Check sheet for the modelled part. Datum: model origin and axes. Units: mm. Face numbers are marked on the shaded views. Give positions to 0.01 mm unless a question says otherwise; leave off trailing zeros. Order: outer loops, then holes, each group sorted by start corner. A loop starts at its lowest first (then second) coordinate and runs counter-clockwise, first axis right, second up. Notation, with made-up numbers: (78, -23.75) -> (82, -23.75) arc R24 ccw to (82, 8.25) -> close; hole circle Ø1 at (22, 44.5). An arc over 180 degrees is marked (long way). Write each question's results on one line, items separated by ' | '.
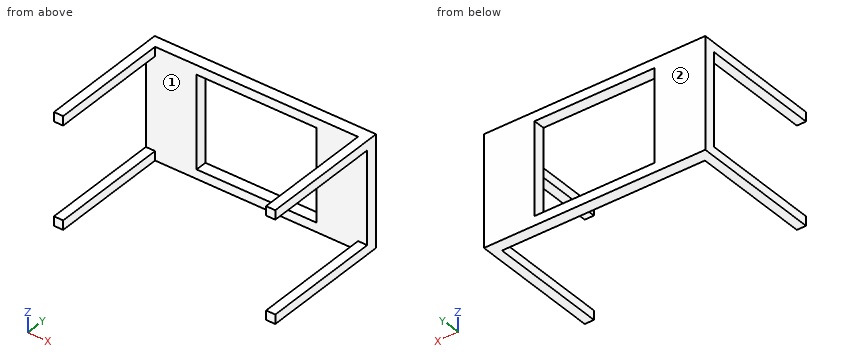
from build123d import *

# Parameters (mm, degrees)
F0_W     = 1219.2
F0_H     = 609.6
F1_DEPTH = 63.5
F2_W     = 660.4
F2_H     = 508
F3_DEPTH = 114.3
F4_W     = 50.8
F4_H     = 50.8
F5_DEPTH = 660.4


with BuildPart() as f1:
    # F0 (on Front) → F1 (new body)
    with BuildSketch(Plane.XZ):
        with Locations((-609.6, 304.8)):
            Rectangle(F0_W, F0_H)
    extrude(amount=F1_DEPTH)

    # F2 (on face) → F3 (cut)
    with BuildSketch(Plane.XZ.offset(63.5)):
        with Locations((-609.6, 304.8)):
            Rectangle(F2_W, F2_H)
    extrude(amount=-F3_DEPTH, mode=Mode.SUBTRACT)

    # F4 (on face) → F5 (join)
    with BuildSketch(Plane.XZ.offset(63.5)):
        with Locations((-1193.8, 584.2)):
            Rectangle(F4_W, F4_H)
        with Locations((-1193.8, 25.4)):
            Rectangle(F4_W, F4_H)
        with Locations((-25.4, 25.4)):
            Rectangle(F4_W, F4_H)
        with Locations((-25.4, 584.2)):
            Rectangle(F4_W, F4_H)
    extrude(amount=F5_DEPTH)


solid = f1.part
1. Gauge pin test, flat ends, axial feed: pin 1 Ø19 at (y, z) = (-36.5, 301.5) entering from +X; pin 2 Ø8 at (x, z) = (-976, 161) entering from -Y. Record the tip position at first contact, or that the pin passes through.
Verdict:
pin 1: stops at x = 0 | pin 2: stops at y = -63.5
2. Section check D-D on x = -107. Record the cut outline in (y, z), then the cut area to 3 significant figures.
Verdict:
outline: (-63.5, 0) -> (0, 0) -> (0, 609.6) -> (-63.5, 609.6) -> close | area: 38,700 mm^2
3. Section check B-B on y = -223.5. Record the cut outline in (x, z), then the cut area to 3 significant figures.
Verdict:
outline: (-1219.2, 0) -> (-1168.4, 0) -> (-1168.4, 50.8) -> (-1219.2, 50.8) -> close; (-1219.2, 558.8) -> (-1168.4, 558.8) -> (-1168.4, 609.6) -> (-1219.2, 609.6) -> close; (-50.8, 0) -> (0, 0) -> (0, 50.8) -> (-50.8, 50.8) -> close; (-50.8, 558.8) -> (0, 558.8) -> (0, 609.6) -> (-50.8, 609.6) -> close | area: 10,300 mm^2
4. Section check C-C on z = 500. Record the cut outline in (x, y).
Verdict:
outline: (-1219.2, -63.5) -> (-939.8, -63.5) -> (-939.8, 0) -> (-1219.2, 0) -> close; (-279.4, -63.5) -> (0, -63.5) -> (0, 0) -> (-279.4, 0) -> close
5. Material ranges on probe 1 along X at (y, z) = (-46.5, 121.5); probe 2 along X at (y, z) = (-244.5, 582.5); probe 3 along Z at (x, y) = (-468, -59.5), recorded low to high. Write a range as from..to.
Verdict:
probe 1: x = -1219.2..-939.8, -279.4..0 | probe 2: x = -1219.2..-1168.4, -50.8..0 | probe 3: z = 0..50.8, 558.8..609.6
6. Mould release check, pull along X, two halves, no side actions. Record for the marked faces 1 and 2: +X half, -X half, draft (parallel to the pull), parting line (faces both ways), or undercut.
Verdict:
face 1: undercut | face 2: draft
7. Section check A-A on x = -781. Record the cut outline in (y, z), then the cut area to 3 significant figures.
Verdict:
outline: (-63.5, 0) -> (0, 0) -> (0, 50.8) -> (-63.5, 50.8) -> close; (-63.5, 558.8) -> (0, 558.8) -> (0, 609.6) -> (-63.5, 609.6) -> close | area: 6,450 mm^2
